```python
from build123d import *

# Parameters (mm, degrees)
SKETCH1_W           = 2.54
SKETCH1_H           = 10
BOSS_EXTRUDE1_DEPTH = 8.1
SKETCH1_3_W         = 0.8
SKETCH1_3_H         = 0.8
BOSS_EXTRUDE2_DEPTH = 3.5
SKETCH2_W           = 2.54
SKETCH2_H           = 3.3
CUT_EXTRUDE1_DEPTH  = 0.2
CUT_EXTRUDE2_DEPTH  = 6
SKETCH4_W           = 0.8
SKETCH4_H           = 0.8
BOSS_EXTRUDE3_DEPTH = 5
LPATTERN1_COUNT     = 12
LPATTERN1_PITCH     = 2.54
BOSS_EXTRUDE4_DEPTH = 0.9
BOSS_EXTRUDE5_START = -30.48
BOSS_EXTRUDE5_DEPTH = 0.9


with BuildPart() as part:
    # Sketch1 → Boss-Extrude1 (new body)
    with BuildSketch(Plane.XY):
        with Locations((13.97, 3.8)):
            Rectangle(SKETCH1_W, SKETCH1_H)
    extrude(amount=BOSS_EXTRUDE1_DEPTH)

    # Sketch1<3> → Boss-Extrude2 (add)
    with BuildSketch(Plane.XY):
        with Locations((13.97, 0)):
            Rectangle(SKETCH1_3_W, SKETCH1_3_H)
    extrude(amount=-BOSS_EXTRUDE2_DEPTH)

    # Sketch2 → Cut-Extrude1 (cut)
    with BuildSketch(Plane.XY.offset(8.1)):
        with Locations((13.97, 7.15)):
            Rectangle(SKETCH2_W, SKETCH2_H)
    extrude(amount=-CUT_EXTRUDE1_DEPTH, mode=Mode.SUBTRACT)

    # Sketch3 → Cut-Extrude2 (cut)
    with BuildSketch(Plane(origin=(0, 8.8, 0), x_dir=(1, 0, 0), z_dir=(0, 1, 0))):
        Polygon((15.24, -2), (12.7, -2), (12.7, -6), (13.5, -6), (13.5, -6.65), (13.1, -6.65), (13.1, -7.5), (14.84, -7.5), (14.84, -6.65), (14.44, -6.65), (14.44, -6), (15.24, -6), align=None)
    extrude(amount=-CUT_EXTRUDE2_DEPTH, mode=Mode.SUBTRACT)

    # Sketch4 → Boss-Extrude3 (add)
    with BuildSketch(Plane(origin=(0, 2.8, 0), x_dir=(1, 0, 0), z_dir=(0, 1, 0))):
        with Locations((13.97, -4)):
            Rectangle(SKETCH4_W, SKETCH4_H)
    extrude(amount=BOSS_EXTRUDE3_DEPTH)


with BuildPart() as lpattern1_1:
    # LPattern1: pattern copy
    add(part.part.moved(Location(Vector(-1, 0, 0) * (1 * LPATTERN1_PITCH))))


with BuildPart() as lpattern1_2:
    # LPattern1: pattern copy
    add(part.part.moved(Location(Vector(-1, 0, 0) * (2 * LPATTERN1_PITCH))))


with BuildPart() as lpattern1_3:
    # LPattern1: pattern copy
    add(part.part.moved(Location(Vector(-1, 0, 0) * (3 * LPATTERN1_PITCH))))


with BuildPart() as lpattern1_4:
    # LPattern1: pattern copy
    add(part.part.moved(Location(Vector(-1, 0, 0) * (4 * LPATTERN1_PITCH))))


with BuildPart() as lpattern1_5:
    # LPattern1: pattern copy
    add(part.part.moved(Location(Vector(-1, 0, 0) * (5 * LPATTERN1_PITCH))))


with BuildPart() as lpattern1_6:
    # LPattern1: pattern copy
    add(part.part.moved(Location(Vector(-1, 0, 0) * (6 * LPATTERN1_PITCH))))


with BuildPart() as lpattern1_7:
    # LPattern1: pattern copy
    add(part.part.moved(Location(Vector(-1, 0, 0) * (7 * LPATTERN1_PITCH))))


with BuildPart() as lpattern1_8:
    # LPattern1: pattern copy
    add(part.part.moved(Location(Vector(-1, 0, 0) * (8 * LPATTERN1_PITCH))))


with BuildPart() as lpattern1_9:
    # LPattern1: pattern copy
    add(part.part.moved(Location(Vector(-1, 0, 0) * (9 * LPATTERN1_PITCH))))


with BuildPart() as lpattern1_10:
    # LPattern1: pattern copy
    add(part.part.moved(Location(Vector(-1, 0, 0) * (10 * LPATTERN1_PITCH))))


with BuildPart() as lpattern1_11:
    # LPattern1: pattern copy
    add(part.part.moved(Location(Vector(-1, 0, 0) * (11 * LPATTERN1_PITCH))))


with BuildPart() as part_1:
    add(part.part)

    # Sketch5 → Boss-Extrude4 (add)
    with BuildSketch(Plane(origin=(15.24, 0, 0), x_dir=(0, 0, -1), z_dir=(1, 0, 0))):
        Polygon((-8.1, -1.2), (0, -1.2), (0, 8.8), (-7.9, 8.8), (-7.9, 5.5), (-8.1, 5.5), align=None)
    extrude(amount=BOSS_EXTRUDE4_DEPTH)


with BuildPart() as body_13:
    # Sketch5<2> → Boss-Extrude5 (new body)
    with BuildSketch(Plane(origin=(15.24, 0, 0), x_dir=(0, 0, -1), z_dir=(1, 0, 0)).offset(BOSS_EXTRUDE5_START)):
        Polygon((-8.1, -1.2), (0, -1.2), (0, 8.8), (-7.9, 8.8), (-7.9, 5.5), (-8.1, 5.5), align=None)
    extrude(amount=-BOSS_EXTRUDE5_DEPTH)


with BuildPart() as lpattern1_1_1:
    add(lpattern1_1.part)

    # Combine1: union LPattern1_2, LPattern1_3, LPattern1_4, LPattern1_5, LPattern1_6, LPattern1_7, LPattern1_8, LPattern1_9, LPattern1_10, LPattern1_11, part, body 13
    add(lpattern1_2.part)
    add(lpattern1_3.part)
    add(lpattern1_4.part)
    add(lpattern1_5.part)
    add(lpattern1_6.part)
    add(lpattern1_7.part)
    add(lpattern1_8.part)
    add(lpattern1_9.part)
    add(lpattern1_10.part)
    add(lpattern1_11.part)
    add(part_1.part)
    add(body_13.part)


solid = lpattern1_1_1.part
```
Can you work these out from the model? Positions are in its coordinate system, mm. A direction names the side the tool comes from. Coordinates: 2 decimals unless noted, no trailing zeros. Loops run counter-clockwise (first coordinate to the right, second up) from the corner with the lowest first, then second, coordinate; pieces in that order, holes last.
1) Imagine slicing it at B-B on z = 5.5. List the corners of the cut face in (x, y) for me, plus the area to 3 significant figures.
2) For pin 1 (1.3 mm diameter, centred on x = -7.5, y = 4.5, fed in from -Z); pin 2 (0.9 mm diameter, centred on x = 14, z = -1, fed in from -Y); pin 3 (0.9 mm diameter, centred on x = -14, z = 4, fed in from +Y), each with a flat end and sliding along its axis, tell me the tip position at first contact or that it passes through.
3) Thinking about a two-plate mould opening in X: for faces 1 (the flat face through (-1, 6, 7.5)), 2 (the flat face through (6.3, 5.3, 3.6)), 3 (the flat face through (0, 2, 8.1)), which applies, pulls with the +X half, pulls with the -X half, needs draft (parallel to the pull), parting line crosses it, or undercut?
4) Which directions (+Z, -Z, +X, -X, +Y, -Y) give clear straight access to the entire face, cutting with the end or side of a thin tool? Please do faces 4 (the flat face through (9, 6, 7.5)), 5 (the flat face through (-11.4, -0.4, -1.7)), 6 (the flat face through (9, 0.4, -2)).
5) I need wall thicknesses on probe 1 along Z at (x, y) = (3.5, 6); probe 2 along X at (y, z) = (8, 4.25); probe 3 along Z at (x, y) = (-5, 8.25). Which ranges of each line are inside material? Lowest first, please.
6) Imagine slicing it at A-A on y = 4.25. State how many separate pieces and enclosed holes the cut face has, plus the area to 3 significant figures.
Completed:
1. outline: (-16.14, -1.2) - (16.14, -1.2) - (16.14, 8.8) - (15.24, 8.8) - (15.24, 2.8) - (-15.24, 2.8) - (-15.24, 8.8) - (-16.14, 8.8) - close
1. area: 140 mm2
2. pin 1: stops at z = 0
2. pin 2: stops at y = -0.4
2. pin 3: stops at y = 7.8
3. face 1: undercut
3. face 2: undercut
3. face 3: needs draft
4. face 4: +Y
4. face 5: -Z, +X, -X, -Y
4. face 6: -Z, +X, -X, +Y
5. probe 1: z = 0 to 2, 3.6 to 4.4, 7.5 to 7.9
5. probe 2: x = -16.14 to -15.24, 15.24 to 16.14
5. probe 3: z = 0 to 2, 6 to 7.9
6. separate pieces: 13
6. enclosed holes: 1
6. area: 122 mm2
